Geometry check sheet. Reference: drawing and pictorial views, mm from the part's lowest x, y, z. A direction names the side the tool comes from. Give positions to 0.01 mm unless a question says otherwise; leave off trailing zeros. Loops run counter-clockwise (first coordinate to the right, second up) from the corner with the lowest first, then second, coordinate; pieces in that order, holes last. Notation, with made-up numbers: (78.5, 36.25) - (94.5, 36.25) arc R23 cw to (94.5, 75.25) - close; hole circle Ø1 at (69, 44.25). An arc over 180 degrees is marked (long way). Answer in a Markdown table with one row per item. Add a question column.
(1) Go/stop test with flat-tipped pins: P1, Ø3, axis at x = 13, z = 1.5, coming from the +Y side; P2, Ø1, axis at y = 5, z = 4, coming from the -X side; P3, Ø0.6, axis at x = 18, y = 3.5, coming from the +Z side; P4, Ø3, axis at y = 4, z = 4.5, coming from the -X side. Record where each tip stops, or that it passes through.
(2) Draft check along Z on the marked faces 4, 5 and 6. Enter one of: released by +Z, released by -Z, zero draft, split by the parting line, or undercut.
(3) Sectioned sample at A-A on x = 17.5. Enter the section's corners in (y, z) (1 decimal), then the cut area to 3 significant figures.
(4) Sectioned sample at C-C on y = 3. Enter the section's corners in (x, z) (3 decimals).
(5) Sectioned sample at B-B on z = 3. Enter the section's corners in (x, y).
(6) Sectioned sample at D-D on x = 7.5. Enter the section's corners in (y, z), then the cut area to 3 significant figures.
(7) Set-up check for the marked faces 1, 2 and 3: record each of +Z, -Z, +X, -X, +Y, -Y from which the full face is reachable in a straight line by a thin tool's end or side.
(8) Thickness scan on L1, parallel to X at y = 2.45, z = 3.9 (1 decimal); L2, parallel to X at y = 4, z = 0.65; L3, parallel to Z at x = 18, y = 2.7 (3 decimals). Record the ranges inside material, lowest first.
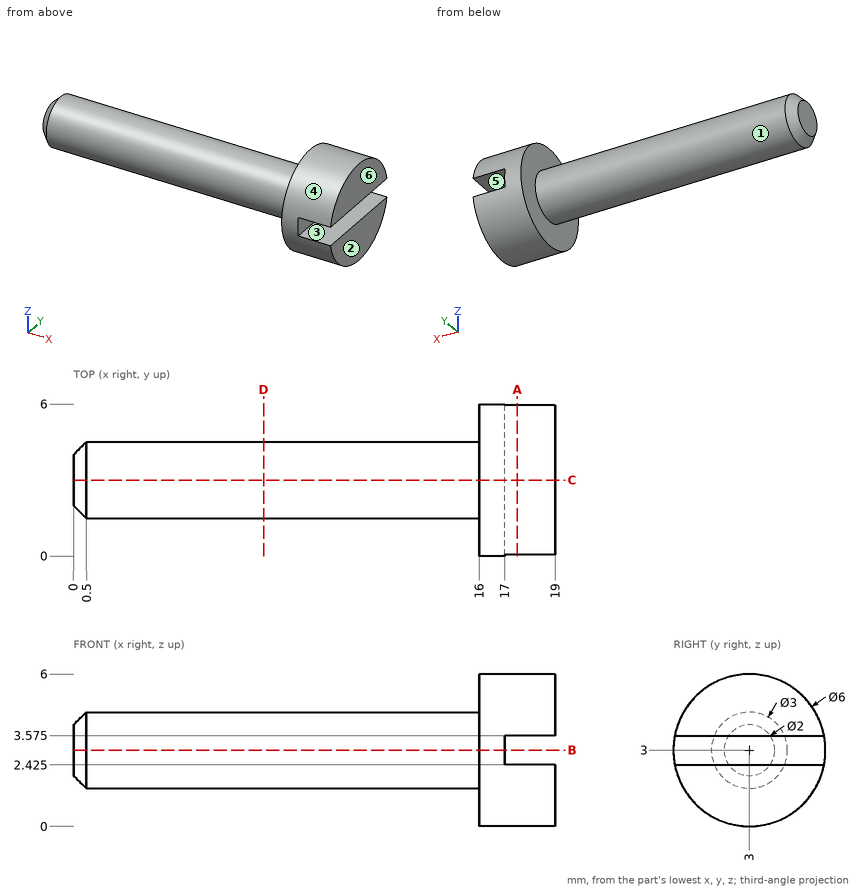
Reply:
| question | item | result |
|---|---|---|
| 1 | P1 | y = 4.5 |
| 1 | P2 | x = 16 |
| 1 | P3 | z = 5.99 |
| 1 | P4 | x = 0 |
| 2 | face 4 | split by the parting line |
| 2 | face 5 | undercut |
| 2 | face 6 | zero draft |
| 3 | outline | (0.1, 2.4) arc R3 ccw to (5.9, 2.4) - close; (0.1, 3.6) - (5.9, 3.6) arc R3 ccw to start |
| 3 | area | 21.4 mm^2 |
| 4 | outline | (0, 2) - (0.5, 1.5) - (16, 1.5) - (16, 0) - (19, 0) - (19, 2.425) - (17, 2.425) - (17, 3.575) - (19, 3.575) - (19, 6) - (16, 6) - (16, 4.5) - (0.5, 4.5) - (0, 4) - close |
| 5 | outline | (0, 2) - (0.5, 1.5) - (16, 1.5) - (16, 0) - (17, 0) - (17, 6) - (16, 6) - (16, 4.5) - (0.5, 4.5) - (0, 4) - close |
| 6 | outline | circle Ø3 at (3, 3) |
| 6 | area | 7.07 mm^2 |
| 7 | face 1 | -X |
| 7 | face 2 | +Z, -Z, +X, +Y, -Y |
| 7 | face 3 | +X, +Y, -Y |
| 8 | L1 | 0.1 to 19 |
| 8 | L2 | 16 to 19 |
| 8 | L3 | 0.015 to 2.425, 3.575 to 5.985 |
